Source: CAD feature listing. Evaluate the final solid. Frame: model axes, mm. A direction names the side the tool comes from. Give positions to 0.01 mm unless a question says otherwise; leave off trailing zeros. Order: outer loops, then holes, each group sorted by start corner. A loop starts at its lowest first (then second) coordinate and runs counter-clockwise, first axis right, second up. Notation, with made-up numbers: (17, -14.75) -> (45, -14.75) arc R23 ccw to (45, -1.75) -> close; hole circle Ø5 at (-35, 72.5). An arc over 180 degrees is marked (long way). Answer in a Markdown table with one row per item.
```python
from build123d import *

# Parameters (mm, degrees)
F0_W     = 76.2
F0_H     = 50.8
F1_DEPTH = 25.4
F2_T     = -2.54
F4_D     = 3.81


with BuildPart() as f1:
    # F0 (on Top) → F1 (new body)
    with BuildSketch(Plane.XY):
        Rectangle(F0_W, F0_H)
    extrude(amount=F1_DEPTH)

    # F2
    f2_openings = [f1.faces().sort_by_distance(p)[0] for p in [
        (0, 0, 25.4),
        (0, -25.4, 12.7),
    ]]
    offset(amount=F2_T, openings=f2_openings)

    # F4 (through all)
    with Locations(Plane(origin=(0, 25.4, 0), x_dir=(-1, 0, 0), z_dir=(0, 1, 0))):
        with Locations((0, 5.159016)):
            Hole(F4_D / 2)


solid = f1.part
```
(1) Section query B-B (y = -19.5). Return the cut outline in (x, z).
A:
| item | result |
|---|---|
| outline | (-38.1, 0) -> (38.1, 0) -> (38.1, 25.4) -> (35.56, 25.4) -> (35.56, 2.54) -> (-35.56, 2.54) -> (-35.56, 25.4) -> (-38.1, 25.4) -> close |
(2) Section query A-A (x = 0). Return the cut outline in (y, z).
A:
| item | result |
|---|---|
| outline | (-25.4, 0) -> (25.4, 0) -> (25.4, 3.25) -> (22.86, 3.25) -> (22.86, 2.54) -> (-25.4, 2.54) -> close; (22.86, 7.06) -> (25.4, 7.06) -> (25.4, 25.4) -> (22.86, 25.4) -> close |
(3) Section query C-C (z = 15.75). Return the cut outline in (x, y), plus the area to 3 significant figures.
A:
| item | result |
|---|---|
| outline | (-38.1, -25.4) -> (-35.56, -25.4) -> (-35.56, 22.86) -> (35.56, 22.86) -> (35.56, -25.4) -> (38.1, -25.4) -> (38.1, 25.4) -> (-38.1, 25.4) -> close |
| area | 439 mm^2 |
(4) Access query for faces 1 (the flat face through (-35.56, -2, 14)), 2 (the flat face through (0, -25.4, 2)). Directions: +Z, -Z, +X, -X, +Y, -Y. A direction counts if a zero-diameter tool reaches every point of the face in a straight line with its end or side. Return the directions, or none.
A:
| item | result |
|---|---|
| face 1 | +Z, -Y |
| face 2 | +Z, -Z, +X, -X, -Y |
(5) Pull-direction query (X, two-part tool) for faces 3 (the flat face through (0, 22.86, 14)), 4 (the flat face through (38.1, 0, 13)), 5 (the flat face through (0, -1, 2.54)), 6 (the flat face through (0, 25, 25.4)); classes: +X half, -X half, draft (parallel to the pull), parting line (faces both ways), or undercut.
A:
| item | result |
|---|---|
| face 3 | undercut |
| face 4 | +X half |
| face 5 | undercut |
| face 6 | draft |
(6) First-contact query: pin 1 Ø14.5 at (x, y) = (-16.5, 4.5) entering from +Z; pin 2 Ø2 at (x, z) = (3.5, 17.5) entering from -Y. Flat tips, straight axial feed; report the tip coordinate or a pass-through.
A:
| item | result |
|---|---|
| pin 1 | stops at z = 2.54 |
| pin 2 | stops at y = 22.86 |
(7) Section query D-D (x = 18). Return the cut outline in (y, z).
A:
| item | result |
|---|---|
| outline | (-25.4, 0) -> (25.4, 0) -> (25.4, 25.4) -> (22.86, 25.4) -> (22.86, 2.54) -> (-25.4, 2.54) -> close |
(8) Ray query, probe 1 along X at (y, z) = (12, 21.5); probe 2 along Z at (x, y) = (0, 24.6); probe 3 along Y at (x, z) = (-9, 18.5). Return the intervals inside material, ascending.
A:
| item | result |
|---|---|
| probe 1 | x = -38.1 to -35.56, 35.56 to 38.1 |
| probe 2 | z = 0 to 3.25, 7.06 to 25.4 |
| probe 3 | y = 22.86 to 25.4 |
